Geometry: see drawing. Coordinates: mm, zero at the bounding-box minimum. Coordinates: 2 decimals unless noted, no trailing zeros. Write each loop counter-clockwise with the first axis right and the second up, starting at its lowest first coordinate (ties: lowest second). Pieces come first, ordered by that corner, then holes. Notation, with made-up numbers: (61, -32) -> (88, -32) arc R7 ccw to (88, -28) -> close; hole circle Ø9 at (66.25, 71). An arc over 180 degrees is marked (long way). Answer as a JSON object with one key per item and string values. Group by question number.
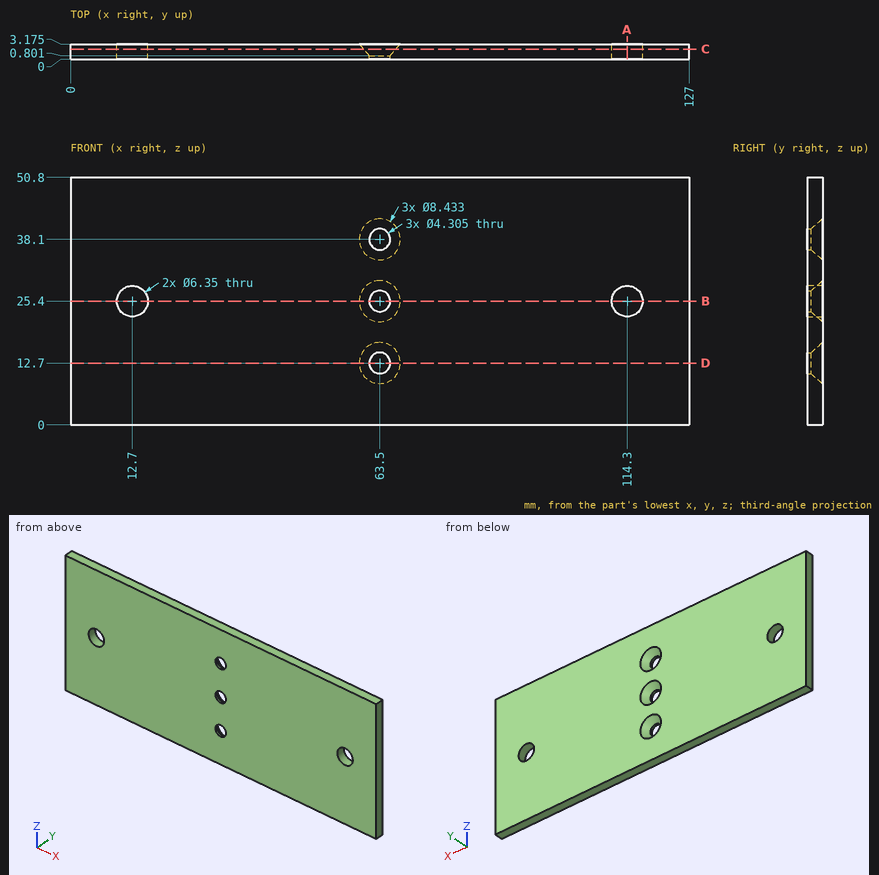
Item 1: Section B-B on z = 25.4. Output: boundary loops of the cut face in (x, y) (1 decimal), then the cut area to 3 significant figures.
Item 2: Section A-A on x = 114.3. Output: boundary loops of the cut face in (y, z) (1 decimal), then the cut area to 3 significant figures.
Item 3: Ray query, L1, parallel to X at y = 0.5, z = 25.4 (1 decimal); L2, parallel to Z at x = 63.5, y = 0.55; L3, parallel to X at y = 0.6, z = 12.7. Return the intervals inside material, ascending. Write a range as [from, to].
Item 4: Contact query for a flat-ended pin moving along its axis: pin 1 (5.5 mm diameter, centred on x = 12.7, z = 25.4, fed in from -Y). Output: stop coordinate, or through.
Item 5: Section D-D on z = 12.7. Output: boundary loops of the cut face in (x, y) (1 decimal), then the cut area to 3 significant figures.
Item 6: Section C-C on y = 2.1. Give the number of separate pieces and of enclosed holes in the cut face, then the cut area to 3 significant figures.
Answer sheet:
{
 "1": {"outline": "(0, 0) -> (9.5, 0) -> (9.5, 3.2) -> (0, 3.2) -> close; (15.9, 0) -> (61.3, 0) -> (61.3, 0.8) -> (59.3, 3.2) -> (15.9, 3.2) -> close; (65.7, 0) -> (111.1, 0) -> (111.1, 3.2) -> (67.7, 3.2) -> (65.7, 0.8) -> close; (117.5, 0) -> (127, 0) -> (127, 3.2) -> (117.5, 3.2) -> close", "area": "344 mm^2"},
 "2": {"outline": "(0, 0) -> (3.2, 0) -> (3.2, 22.2) -> (0, 22.2) -> close; (0, 28.6) -> (3.2, 28.6) -> (3.2, 50.8) -> (0, 50.8) -> close", "area": "141 mm^2"},
 "3": {"L1": "x = [0, 9.5], [15.9, 61.3], [65.7, 111.1], [117.5, 127]", "L2": "z = [0, 10.55], [14.85, 23.25], [27.55, 35.95], [40.25, 50.8]", "L3": "x = [0, 61.35], [65.65, 127]"},
 "4": {"pin 1": "passes through"},
 "5": {"outline": "(0, 0) -> (61.3, 0) -> (61.3, 0.8) -> (59.3, 3.2) -> (0, 3.2) -> close; (65.7, 0) -> (127, 0) -> (127, 3.2) -> (67.7, 3.2) -> (65.7, 0.8) -> close", "area": "385 mm^2"},
 "6": {"separate pieces": "1", "enclosed holes": "5", "area": "6,290 mm^2"}
}
